CAD build for the part. Positions are in the model's coordinates, mm. A direction names the side the tool comes from. Coordinates: 2 decimals unless noted, no trailing zeros. Order: outer loops, then holes, each group sorted by start corner. A loop starts at its lowest first (then second) coordinate and runs counter-clockwise, first axis right, second up. Notation, with made-up numbers: M -7,15 L 4,15 A21 cw 4,27 Z; hole C 64,17.25 d9. An arc over 180 degrees is marked long. Write item = value, one per line.
from build123d import *

# Parameters (mm, degrees)
F1_DEPTH   = 19.05
F4_D       = 7.1374
F4_ON_F2_D = 7.1374


with BuildPart() as f1:
    # F0 (on Right) → F1 (new body, symmetric)
    with BuildSketch(Plane.YZ):
        Polygon((0, 0), (0, 203.2), (-6.3499999233, 203.2), (-6.3499999233, 6.3499999233), (-127, 6.3499999233), (-127, 0), align=None)
    extrude(amount=F1_DEPTH, both=True)

    # F4 (through all)
    with Locations(Plane.XZ.offset(6.3499999233)):
        with Locations((0, 158.7499999233), (0, 120.6499999233), (0, 82.5499999233), (0, 44.4499999233)):
            Hole(F4_D / 2)

    # F4 on F2 (through all)
    with Locations(Plane.XY.offset(6.3499999233)):
        with Locations((0, -44.4499999233), (0, -82.5499999233)):
            Hole(F4_ON_F2_D / 2)


solid = f1.part
(1) Pin check, flat tips, straight feed: pin 1 Ø9.5 at (x, y) = (0, -44.45) entering from +Z; pin 2 Ø10 at (x, z) = (14, 117.5) entering from -Y; pin 3 Ø6.5 at (x, z) = (0, 120.65) entering from -Y. Stop position of each tip, or through.
Evaluation:
pin_1 = 6.35
pin_2 = -6.35
pin_3 = through
(2) Slice it at B-B, the plane x = 0. State how many separate pieces and enclosed holes the cut face has, then the cut area to 3 significant figures.
Evaluation:
separate_pieces = 7
enclosed_holes = 0
area = 1,780 mm²
(3) Slice it at C-C, the plane z = 120.65. Write the cut outline in (x, y).
Evaluation:
outline = M -19.05,-6.35 L -3.57,-6.35 L -3.57,0 L -19.05,0 Z; M 3.57,-6.35 L 19.05,-6.35 L 19.05,0 L 3.57,0 Z
(4) Slice it at D-D, the plane y = -38. Write the cut outline in (x, z).
Evaluation:
outline = M -19.05,0 L 19.05,0 L 19.05,6.35 L -19.05,6.35 Z
(5) Wall check: line 1 (Z direction, x = 0, y = -4); line 2 (Y direction, x = 0, z = 2); line 3 (X direction, y = -4, z = 82). Give the ranges that are in metal, low to high. Write a range as from..to.
Evaluation:
line_1 = 0..40.88, 48.02..78.98, 86.12..117.08, 124.22..155.18, 162.32..203.2
line_2 = -127..-86.12, -78.98..-48.02, -40.88..0
line_3 = -19.05..-3.53, 3.53..19.05
(6) Tool access for faces 1 (the face through (0, -66, 6.35)), 2 (the face through (0, -64, 0)): list every direction of +Z, -Z, +X, -X, +Y, -Y with a clear straight run to the whole face (end or side of a thin tool).
Evaluation:
face_1 = +Z, +X, -X, -Y
face_2 = -Z, +X, -X, +Y, -Y
(7) Slice it at A-A, the plane y = -82.55. Write the cut outline in (x, z).
Evaluation:
outline = M -19.05,0 L -3.57,0 L -3.57,6.35 L -19.05,6.35 Z; M 3.57,0 L 19.05,0 L 19.05,6.35 L 3.57,6.35 Z
(8) Pull direction Y, two halves, no side cores. Call faces 3 (the face through (19.05, -3, 57)), 4 (the face through (0, -6.35, 106)), 5 (the face through (-1.647, -85.716, 3.131)), 6 (the face through (0, 0, 100)): +Y half, -Y half, draft (parallel to the pull), parting line (faces both ways), or undercut.
Evaluation:
face_3 = draft
face_4 = -Y half
face_5 = undercut
face_6 = +Y half
